Autodesk Inventor part; units mm, degrees
ref_plane "YZ Plane" through (0, 0, 0) normal (1, 0, 0) x (0, 1, 0)
ref_plane "XZ Plane" through (0, 0, 0) normal (0, 1, 0) x (-1, 0, 0)
ref_plane "XY Plane" through (0, 0, 0) normal (0, 0, 1) x (1, 0, 0)
sketch "Sketch1" plane through (0, 0, 0) normal (0, 0, 1) x (1, 0, 0)
  circle A0 centre (0, 0) radius 4 construction
  circle A1 centre (-12, 0) radius 2.25
  circle A2 centre (12, 0) radius 2.25
  line L0 (-12, 0) -> (0, 0) construction
  line L1 (12, 0) -> (0, 0) construction
  arc A3 (-13, 5.9161) -> (-13, -5.9161) centre (-12, 0) ccw
  arc A4 (13, -5.9161) -> (13, 5.9161) centre (12, 0) ccw
  line L2 (-13, 5.9161) -> (-1.3333, 7.8881)
  line L3 (1.3333, 7.8881) -> (13, 5.9161)
  line L4 (1.3333, -7.8881) -> (13, -5.9161)
  line L5 (-1.3333, -7.8881) -> (-13, -5.9161)
  arc A5 (1.3333, 7.8881) -> (-1.3333, 7.8881) centre (0, 0) ccw
  arc A6 (-1.3333, -7.8881) -> (1.3333, -7.8881) centre (0, 0) ccw
  circle A7 centre (-12, 0) radius 4.5 construction
  dimension "d0" = 8
  dimension "d2" = 4.5
  dimension "d3" = 8
  dimension "d4" = 12
  dimension "d5" = 9
  dimension "d6" = 6
extrude "Extrusion1" add sketch "Sketch1" along normal blind 6.5
properties part number "y_axis_cap" material "Plywood, Finish"
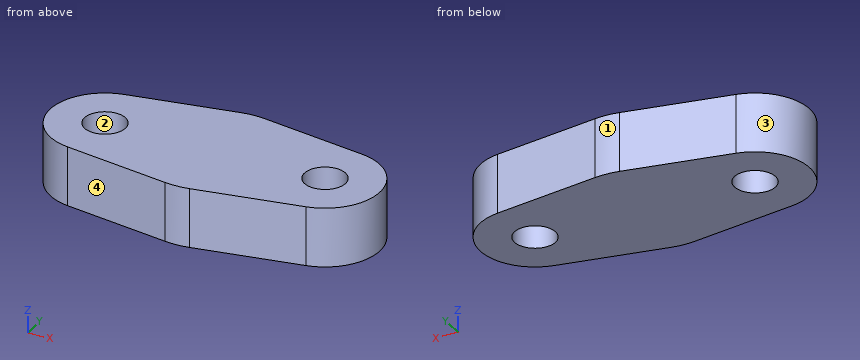
CAD build for the part. Positions are in the model's coordinates, mm. Face numbers are marked on the shaded views. Give positions to 0.01 mm unless a question says otherwise; leave off trailing zeros. Write each loop counter-clockwise with the first axis right and the second up, starting at its lowest first coordinate (ties: lowest second). Pieces come first, ordered by that corner, then holes. Notation, with made-up numbers: M 56,34 L 109,34 A20 ccw 109,40 Z; hole C -31.5,-12 d4. An arc over 180 degrees is marked long. Return JSON: item names as keys, results as strings. Group by question number.
(1) Flat gauge pins, fed straight in: pin 1 Ø2.5 at (x, y) = (-12, 0) entering from -Z; pin 2 Ø1.5 at (x, z) = (4, 5) entering from +Y; pin 3 Ø1 at (y, z) = (6, 3.5) entering from -X; pin 4 Ø1 at (y, z) = (4, 1.5) entering from -X. Where does each tip first touch, or does it go through?
(2) Mould opens along Y. For the marked faces 1, 2, 3 and 4 say: pulls with the +Y half, pulls with the -Y half, needs draft (parallel to the pull), parting line crosses it, or undercut.
(3) Band-saw the part on B-B (z = 2). Give the cut face in (x, y), and give its area (3 significant figures).
(4) Band-saw the part on D-D (x = 2.5). Give the cut face in (y, z), and give its area (4 significant figures).
(5) Band-saw the part on C-C (x = 12). Give the cut face in (y, z).
(6) Band-saw the part on A-A (y = 0). Give the cut face in (x, z), and give its area (4 significant figures).
(7) Drill centre lines: L1, parallel to X at y = -1.5, z = 1; L2, parallel to X at y = 1.75, z = 2.5; L3, parallel to Y at x = -12, z = 2.5. Where is each one in solid material? Low to high. Write a range as [from, to].
Entries:
{
 "1": {"pin 1": "passes through", "pin 2": "stops at y = 7.56", "pin 3": "stops at x = -14.4", "pin 4": "stops at x = -16.87"},
 "2": {"face 1": "pulls with the +Y half", "face 2": "undercut", "face 3": "parting line crosses it", "face 4": "pulls with the -Y half"},
 "3": {"outline": "M -13,-5.92 L -1.33,-7.89 A8 ccw 1.33,-7.89 L 13,-5.92 A6 ccw 13,5.92 L 1.33,7.89 A8 ccw -1.33,7.89 L -13,5.92 A6 ccw Z; hole C -12,0 d4.5; hole C 12,0 d4.5", "area": "422 mm^2"},
 "4": {"outline": "M -7.69,0 L 7.69,0 L 7.69,6.5 L -7.69,6.5 Z", "area": "100.0 mm^2"},
 "5": {"outline": "M -6.09,0 L -2.25,0 L -2.25,6.5 L -6.09,6.5 Z; M 2.25,0 L 6.09,0 L 6.09,6.5 L 2.25,6.5 Z"},
 "6": {"outline": "M -18,0 L -14.25,0 L -14.25,6.5 L -18,6.5 Z; M -9.75,0 L 9.75,0 L 9.75,6.5 L -9.75,6.5 Z; M 14.25,0 L 18,0 L 18,6.5 L 14.25,6.5 Z", "area": "175.5 mm^2"},
 "7": {"L1": "x = [-17.81, -13.68], [-10.32, 10.32], [13.68, 17.81]", "L2": "x = [-17.74, -13.41], [-10.59, 10.59], [13.41, 17.74]", "L3": "y = [-6.09, -2.25], [2.25, 6.09]"}
}
